Can you work these out from the drawing? Everything is in mm from the part's minimum corner. A direction names the side the tool comes from. Round coordinates to 2 decimals unless told otherwise and drop trailing zeros. Loops run counter-clockwise (first coordinate to the right, second up) from the corner with the lowest first, then second, coordinate; pieces in that order, holes last. Notation, with made-up numbers: M 74.25,56.5 L 103.25,56.5 A30 cw 103.25,91.5 Z; hole C 49,14.25 d8. An arc over 180 degrees is marked long. Use a Markdown table: item, result.
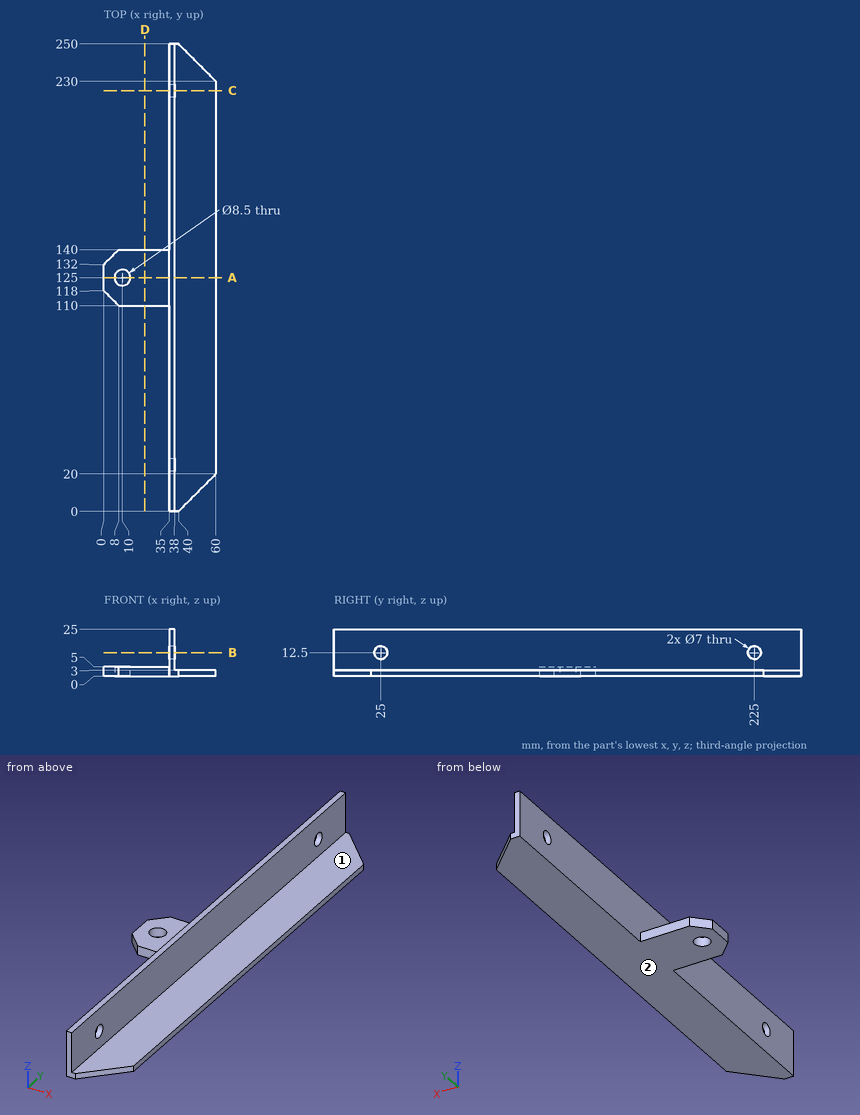
1. For pin 1 Ø11 at (y, z) = (25, 12.5) entering from +X; pin 2 Ø7 at (x, y) = (10, 125) entering from -Z; pin 3 Ø1.5 at (y, z) = (183.5, 18.5) entering from -X; pin 4 Ø1.5 at (x, z) = (22, 1.5) entering from -Y, each with a flat end and sliding along its axis, tell me the tip position at first contact or that it passes through.
Answer sheet:
| item | result |
|---|---|
| pin 1 | x = 38 |
| pin 2 | through |
| pin 3 | x = 35 |
| pin 4 | y = 110 |
2. Imagine slicing it at A-A, the plane y = 125. Write out the boundary of the cut face in (x, z), then the cut area to 4 significant figures.
Answer sheet:
| item | result |
|---|---|
| outline | M 0,0 L 5.75,0 L 5.75,5 L 0,5 Z; M 14.25,0 L 60,0 L 60,3 L 38,3 L 38,25 L 35,25 L 35,5 L 14.25,5 Z |
| area | 273.5 mm2 |
3. Which directions (+Z, -Z, +X, -X, +Y, -Y) give clear straight access to the entire face, cutting with the end or side of a thin tool? Please do the marked faces 1 and 2.
Answer sheet:
| item | result |
|---|---|
| face 1 | +Z, +X, +Y, -Y |
| face 2 | -Z, +X, -X, +Y, -Y |
4. I need wall thicknesses on probe 1 along Y at (x, z) = (35.8, 12.5); probe 2 along Y at (x, z) = (10, 3.8); probe 3 along Z at (x, y) = (37, 225). Which ranges of each line are inside material? Lowest first, please. Write a range as from..to.
Answer sheet:
| item | result |
|---|---|
| probe 1 | 0..21.5, 28.5..221.5, 228.5..250 |
| probe 2 | 110..120.75, 129.25..140 |
| probe 3 | 0..9, 16..25 |
5. Imagine slicing it at B-B, the plane z = 12.5. Write out the boundary of the cut face in (x, y).
Answer sheet:
| item | result |
|---|---|
| outline | M 35,0 L 38,0 L 38,21.5 L 35,21.5 Z; M 35,28.5 L 38,28.5 L 38,221.5 L 35,221.5 Z; M 35,228.5 L 38,228.5 L 38,250 L 35,250 Z |
6. Imagine slicing it at D-D, the plane x = 22. Write out the boundary of the cut face in (y, z), then the cut area to 3 significant figures.
Answer sheet:
| item | result |
|---|---|
| outline | M 110,0 L 140,0 L 140,5 L 110,5 Z |
| area | 150 mm2 |
7. Imagine slicing it at C-C, the plane y = 225. Write out the boundary of the cut face in (x, z).
Answer sheet:
| item | result |
|---|---|
| outline | M 35,0 L 60,0 L 60,3 L 38,3 L 38,9 L 35,9 Z; M 35,16 L 38,16 L 38,25 L 35,25 Z |
